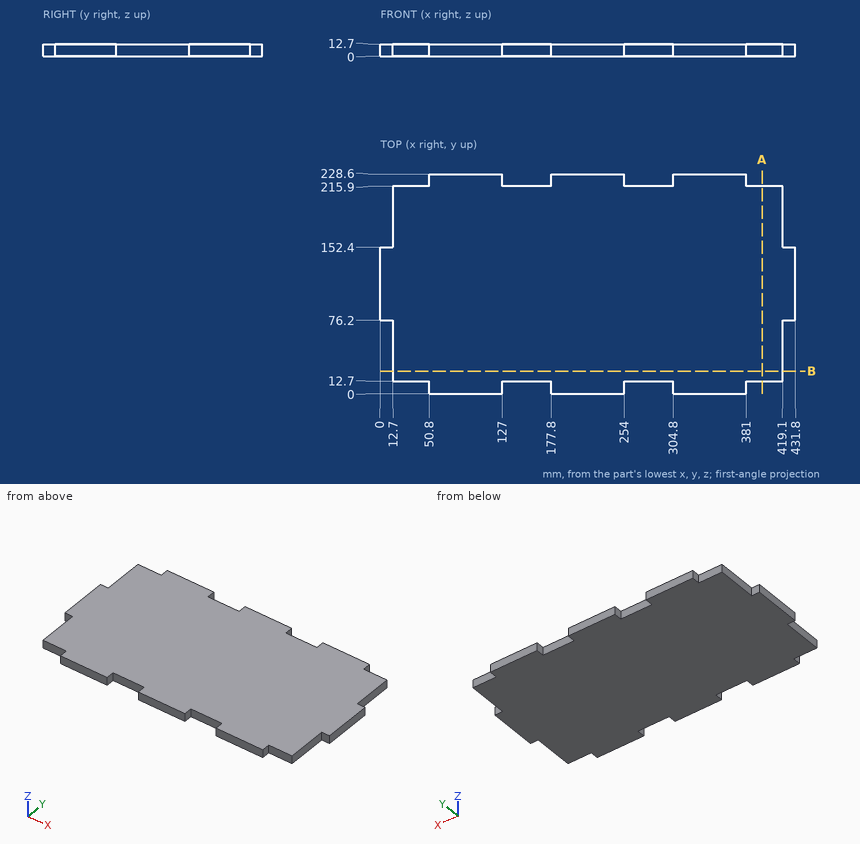
Design review of the part shown in the three views and the two pictorial views. Dimensions are in mm from the part's minimum x, y and z. Coordinates: 2 decimals unless noted, no trailing zeros. Loops run counter-clockwise (first coordinate to the right, second up) from the corner with the lowest first, then second, coordinate; pieces in that order, holes last. Notation, with made-up numbers: (-2, -8) -> (9, -8) arc R20 cw to (9, 4) -> close; hole circle Ø11 at (-19.75, 81). An arc over 180 degrees is marked (long way). Answer as CSV lines item,"result".
Item 1: For L1, parallel to X at y = 11.5, z = 5.25; L2, parallel to X at y = 195, z = 6.25; L3, parallel to Y at x = 301, z = 5.25, list the stretches that pass through material, from the lowest coordinate up.
Results below:
L1,"x = 50.8 to 127, 177.8 to 254, 304.8 to 381"
L2,"x = 12.7 to 419.1"
L3,"y = 12.7 to 215.9"
Item 2: Take a section at A-A, the plane x = 397.5. State the section outline as (y, z) points.
Results below:
outline,"(12.7, 0) -> (215.9, 0) -> (215.9, 12.7) -> (12.7, 12.7) -> close"
Item 3: Take a section at B-B, the plane y = 23.5. State the section outline as (x, z) points.
Results below:
outline,"(12.7, 0) -> (419.1, 0) -> (419.1, 12.7) -> (12.7, 12.7) -> close"
Item 4: Insertion check: pin 1 (6.5 mm diameter, centred on x = 142.5, z = 6.5, fed in from +Y); pin 2 (2 mm diameter, centred on x = 64, y = 197.5, fed in from -Z); pin 3 (6.5 mm diameter, centred on y = 44.5, z = 7, fed in from -X); pin 4 (4 mm diameter, centred on y = 225, z = 4, fed in from -X). Each pin has a flat end and moves straight along its axis. Give the tip position at first contact, or say it passes through.
Results below:
pin 1,"stops at y = 215.9"
pin 2,"stops at z = 0"
pin 3,"stops at x = 12.7"
pin 4,"stops at x = 50.8"
